Autodesk Inventor part; units mm, degrees
ref_plane "YZ Plane" through (0, 0, 0) normal (1, 0, 0) x (0, 1, 0)
ref_plane "XZ Plane" through (0, 0, 0) normal (0, 1, 0) x (-1, 0, 0)
ref_plane "XY Plane" through (0, 0, 0) normal (0, 0, 1) x (1, 0, 0)
sketch "Sketch1" plane through (0, 0, 0) normal (0, 1, 0) x (-1, 0, 0)
  line L0 (11, 7) -> (-10.5, 7)
  line L1 (-10.5, 7) -> (-10.5, -7)
  line L2 (-10.5, -7) -> (11, -7)
  line L3 (11, -7) -> (11, 7)
  point P0 (0, 0)
  dimension "d0" = 21.5
  dimension "d1" = 14
  dimension "d2" = 7
  dimension "d3" = 11
extrude "Extrusion1" add sketch "Sketch1" along normal blind 10
fillet "Fillet1" radius 1 4 edges at (10.5, 5, 7) (10.5, 5, -7) (-11, 5, -7) (-11, 5, 7)
shell "Shell1" thickness 1.5 removed faces 1 at (3, 0, 2.3333)
sketch "Sketch2" plane through (0, 10, 0) normal (0, 1, 0) x (1, 0, 0)
  line L0 (-6.25, 3) -> (5.75, 3)
  line L1 (5.75, 3) -> (5.75, -3)
  line L2 (5.75, -3) -> (-6.25, -3)
  line L3 (-6.25, -3) -> (-6.25, 3)
  line L4 (10.5, -6) -> (10.5, 6)
  point P0 (0, 0)
  dimension "d8" = 6
  dimension "d9" = 12
  dimension "d10" = 3
  dimension "d33" = 4.75
extrude "Extrusion2" cut sketch "Sketch2" against normal blind 10
sketch "Sketch4" plane through (0, 0, 0) normal (0, -1, 0) x (1, 0, 0)
  line L0 (10.25, 4) -> (9.25, 4)
  line L1 (9.25, 4) -> (9.25, -4)
  line L2 (9.25, -4) -> (10.25, -4)
  line L3 (10.25, -4) -> (10.25, 4)
  line L4 (10.5, 6) -> (10.5, -6)
  line L5 (-9.5, 5.5) -> (9, 5.5)
  line L6 (-9.75, 4) -> (-10.75, 4)
  line L7 (-10.75, 4) -> (-10.75, -4)
  line L8 (-10.75, -4) -> (-9.75, -4)
  line L9 (-9.75, -4) -> (-9.75, 4)
  line L10 (-11, -6) -> (-11, 6)
  line L11 (9, -5.5) -> (-9.5, -5.5)
  line L12 (-10, 7) -> (9.5, 7)
  line L13 (9.5, -7) -> (-10, -7)
  point P0 (0, 0)
  dimension "d20" = 1
  dimension "d23" = 1
  dimension "d24" = 8
  dimension "d25" = 0.25
  dimension "d29" = 3
  dimension "d30" = 3
  dimension "d31" = 8
  dimension "d32" = 0.25
extrude "Extrusion3" add sketch "Sketch4" along normal blind 1.5
sketch "Sketch5" plane through (-10, 0, 7) normal (0, 0, 1) x (1, 0, 0)
  line L0 (0, 0) -> (19.5, 0)
  line L1 (5.75, 2) -> (13.75, 2)
  line L2 (13.75, 2) -> (13.75, 0)
  line L3 (13.75, 0) -> (5.75, 0)
  line L4 (5.75, 0) -> (5.75, 2)
  line L5 (-1, 10) -> (-1, 0)
  point P0 (10, 0)
  dimension "d34" = 8
  dimension "d35" = 2
  dimension "d36" = 6.75
extrude "Extrusion4" cut sketch "Sketch5" against normal blind 10
properties part number "Black_Keyboard_Button_Base"
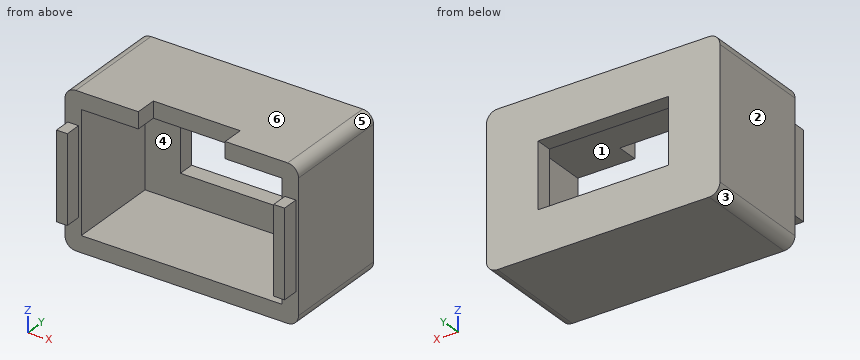
Verification items for the finished model (mm, model axes). Face numbers are marked on the shaded views. A direction names the side the tool comes from. Give positions to 0.01 mm unless a question says otherwise; leave off trailing zeros. Loops run counter-clockwise (first coordinate to the right, second up) from the corner with the lowest first, then second, coordinate; pieces in that order, holes last.
1) Depth check by flat-ended pin: pin 1 Ø1.2 at (y, z) = (-0.5, 0.5) entering from +X; pin 2 Ø1.2 at (y, z) = (-1, -1.5) entering from +X; pin 3 Ø6 at (x, z) = (-4.5, -3.5) entering from -Y; pin 4 Ø0.5 at (x, y) = (-10, -0.5) entering from -Z. Enter the tip coordinate at first touch or a pass-through.
2) Sectioned sample at A-A, the plane x = 5. Enter the section's corners in (y, z), then the cut area to 3 significant figures.
3) Thickness scan on line 1 along X through (y, z) = (4.5, -5); line 2 along Z through (x, y) = (4.75, 9.5); line 3 along Z through (x, y) = (6.5, 1.25). Record the ranges inside material, lowest first.
4) Set-up check for the marked faces 1 and 2: record each of +Z, -Z, +X, -X, +Y, -Y from which the full face is reachable in a straight line by a thin tool's end or side.
5) Draft check along X on the marked faces 3, 4, 5 and 6. Enter one of: pulls with the +X half, pulls with the -X half, needs draft (parallel to the pull), parting line crosses it, or undercut.
6) Sectioned sample at B-B, the plane y = 5.25. Enter the section's corners in (x, z), then the cut area to 3 significant figures.
7) Sectioned sample at C-C, the plane z = -0.5. Enter the section's corners in (x, y).
8) Sectioned sample at D-D, the plane z = -4.75. Enter the section's corners in (x, y), then the cut area to 4 significant figures.
Answers:
1. pin 1: stops at x = 10.5
1. pin 2: stops at x = 10.25
1. pin 3: stops at y = 0
1. pin 4: stops at z = -4
2. outline: (0, -7) - (10, -7) - (10, -3) - (8.5, -3) - (8.5, -5.5) - (0, -5.5) - close; (0, 5.5) - (8.5, 5.5) - (8.5, 3) - (10, 3) - (10, 7) - (0, 7) - close
2. area: 37.5 mm2
3. line 1: x = -11 to -9.5, 9 to 10.5
3. line 2: z = -7 to -3, 3 to 7
3. line 3: z = -7 to -5.5, 5.5 to 7
4. face 1: -Y
4. face 2: +Z, -Z, -X, +Y, -Y
5. face 3: pulls with the -X half
5. face 4: undercut
5. face 5: pulls with the +X half
5. face 6: needs draft
6. outline: (-11, -6) arc R1 ccw to (-10, -7) - (9.5, -7) arc R1 ccw to (10.5, -6) - (10.5, 6) arc R1 ccw to (9.5, 7) - (-10, 7) arc R1 ccw to (-11, 6) - close; hole (-9.5, -5.5) - (9, -5.5) - (9, 5.5) - (-9.5, 5.5) - close
6. area: 96.6 mm2
7. outline: (-11, 0) - (-10.75, 0) - (-10.75, -1.5) - (-9.75, -1.5) - (-9.75, 0) - (-9.5, 0) - (-9.5, 8.5) - (-6.25, 8.5) - (-6.25, 10) - (-11, 10) - close; (5.75, 8.5) - (9, 8.5) - (9, 0) - (9.25, 0) - (9.25, -1.5) - (10.25, -1.5) - (10.25, 0) - (10.5, 0) - (10.5, 10) - (5.75, 10) - close
8. outline: (-11, 0) - (-9.5, 0) - (-9.5, 8.5) - (9, 8.5) - (9, 0) - (10.5, 0) - (10.5, 10) - (-11, 10) - close
8. area: 57.75 mm2
